```python
from build123d import *

# Parameters (mm, degrees)
BOSS_EXTRUDE1_DEPTH = 3.175
SKETCH3_R           = 2.1
CUT_EXTRUDE1_DEPTH  = 10


with BuildPart() as part:
    # Sketch1 → Boss-Extrude1 (new body)
    with BuildSketch(Plane.XY):
        with BuildLine():
            Line((-105, 44.736808962), (-101.95, 14.38969213))
            ThreePointArc((-101.95, 14.38969213), (-119.402255024, -6.962562893), (-98.05, -24.414817917))
            Line((-98.05, -24.414817917), (-95, -54.761934749))
            ThreePointArc((-95, -54.761934749), (0, -50), (95, -54.761934749))
            Line((95, -54.761934749), (98, -24.912311636))
            ThreePointArc((98, -24.912311636), (80.100251258, -3.012562893), (102, 14.887185849))
            Line((102, 14.887185849), (105, 44.736808962))
            ThreePointArc((105, 44.736808962), (0, 50), (-105, 44.736808962))
        make_face()
        with BuildLine():
            Line((-14.021567416, 1.25), (-9.921567416, 1.25))
            ThreePointArc((-9.921567416, 1.25), (0, 10), (9.921567416, 1.25))
            Line((9.921567416, 1.25), (14.021567416, 1.25))
            Line((14.021567416, 1.25), (14.021567416, -1.25))
            Line((14.021567416, -1.25), (9.921567416, -1.25))
            ThreePointArc((9.921567416, -1.25), (0, -10), (-9.921567416, -1.25))
            Line((-9.921567416, -1.25), (-14.021567416, -1.25))
            Line((-14.021567416, -1.25), (-14.021567416, 1.25))
        make_face(mode=Mode.SUBTRACT)
    extrude(amount=BOSS_EXTRUDE1_DEPTH)

    # Sketch3 → Cut-Extrude1 (cut)
    with BuildSketch(Plane.XY.offset(3.175)):
        with Locations((-94.396840498, 39.233865601)):
            Circle(SKETCH3_R)
        with Locations((-93.239490742, 27.289806762)):
            Circle(SKETCH3_R)
        with Locations((-86.896840498, -35.390192182)):
            Circle(SKETCH3_R)
        with Locations((-85.739490742, -47.334251021)):
            Circle(SKETCH3_R)
        with Locations((85.70397559, -47.259048155)):
            Circle(SKETCH3_R)
        with Locations((86.946610528, -35.3235608)):
            Circle(SKETCH3_R)
        with Locations((93.20397559, 27.365009628)):
            Circle(SKETCH3_R)
        with Locations((94.446610528, 39.300496983)):
            Circle(SKETCH3_R)
    extrude(amount=-CUT_EXTRUDE1_DEPTH, mode=Mode.SUBTRACT)


solid = part.part
```
Part model, mm, in its own coordinate system. A direction names the side the tool comes from. Coordinates: 2 decimals unless noted, no trailing zeros. Order: outer loops, then holes, each group sorted by start corner. A loop starts at its lowest first (then second) coordinate and runs counter-clockwise, first axis right, second up. Notation, with made-up numbers: (3.25, 77.25) -> (39.25, 77.25) arc R35 ccw to (39.25, 112.25) -> close; hole circle Ø8 at (88.25, 76). An arc over 180 degrees is marked (long way). Put each result on its own line as item: value. Start each with the question number.
(1) Band-saw the part on C-C (x = -60). Give the cut face in (y, z) (3 decimals).
(2) Which spindle directions (+Z, -Z, +X, -X, +Y, -Y) get a long thin tool onto all of the face, cutting with end or side? Do faces 1 (the face through (0, -10, 2)), 2 (the face through (-9, 10, 0)). Say none if no direction does.
(3) Band-saw the part on A-A (z = 2.65). Count the separate pieces of the cut face and the enclosed holes in it, then the cut area to 3 significant figures.
(4) Probe line 1 along X through (y, z) = (-48.5, 1.1); line 2 along Y through (x, z) = (1, 1.3); line 3 along Y through (x, z) = (-94, 0.2). List the from-to ranges inside material, lowest first. Write a range as [from, to].
(5) Band-saw the part on B-B (x = 75.5). Give the cut face in (y, z) (3 decimals).
(6) Pin check, flat tips, straight feed: pin 1 Ø1 at (x, z) = (-18, 1) entering from -Y; pin 2 Ø1 at (y, z) = (33.5, 2.5) entering from -X; pin 3 Ø1.2 at (y, z) = (0, 2) entering from -X; pin 4 Ø6.5 at (x, y) = (86.95, -35.32) entering from +Z (3 decimals). Stop position of each tip, or through.
(7) Mould opens along X. For faces 3 (the face through (-1, -50, 2)), 4 (the face through (1, 50, 2)), 5 (the face through (-9, 10, 3.175)) say: pulls with the +X half, pulls with the -X half, needs draft (parallel to the pull), parting line crosses it, or undercut.
Determined:
1. outline: (-51.897, 0) -> (48.284, 0) -> (48.284, 3.175) -> (-51.897, 3.175) -> close
2. face 1: +Z, -Z
2. face 2: -Z, +X, -X, +Y, -Y
3. separate pieces: 1
3. enclosed holes: 9
3. area: 19,600 mm²
4. line 1: x = [-95.63, -87.49], [-83.99, 84.01], [87.4, 95.63]
4. line 2: y = [-50, -9.95], [9.95, 50]
4. line 3: y = [-54.66, 25.33], [29.25, 37.17], [41.3, 45.78]
5. outline: (-53.005, 0) -> (47.282, 0) -> (47.282, 3.175) -> (-53.005, 3.175) -> close
6. pin 1: stops at y = -50.18
6. pin 2: stops at x = -103.92
6. pin 3: stops at x = -118.99
6. pin 4: stops at z = 3.175
7. face 3: undercut
7. face 4: parting line crosses it
7. face 5: needs draft
